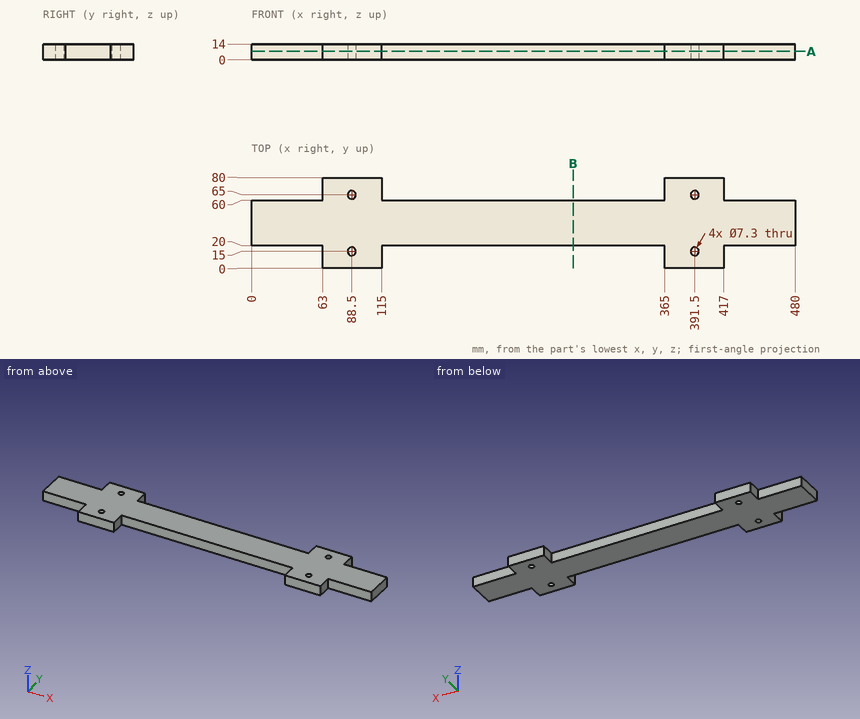
Geometry check sheet. Reference: drawing and pictorial views, mm from the part's lowest x, y, z. Round coordinates to 2 decimals unless told otherwise and drop trailing zeros. Order: outer loops, then holes, each group sorted by start corner. A loop starts at its lowest first (then second) coordinate and runs counter-clockwise, first axis right, second up. Notation, with made-up numbers: (21.25, -4) -> (31.25, -4) arc R29 ccw to (31.25, 25) -> close; hole circle Ø9 at (-0.75, -28). An arc over 180 degrees is marked (long way). One line per item, written item: value. Start each with the question number.
Q1. Gauge pin test, flat ends, axial feed: pin 1 Ø7 at (y, z) = (11.5, 4.5) entering from -X; pin 2 Ø11.5 at (x, y) = (391.5, 15) entering from +Z; pin 3 Ø2 at (x, z) = (215.5, 2) entering from -Y; pin 4 Ø7 at (y, z) = (14, 4) entering from +X. Record the tip position at first contact, or that the pin passes through.
Q2. Cross-section at A-A (z = 7.5). Record the boundary of the cut face in (x, y), and give its area (3 significant figures).
Q3. Thickness scan on line 1 (Y direction, x = 88.5, z = 11); line 2 (Y direction, x = 91, z = 8.75); line 3 (Y direction, x = 161, z = 4.25). Record the ranges inside material, lowest first.
Q4. Cross-section at B-B (x = 284). Record the boundary of the cut face in (y, z).
Completed:
1. pin 1: stops at x = 63
1. pin 2: stops at z = 14
1. pin 3: stops at y = 20
1. pin 4: stops at x = 417
2. outline: (0, 20) -> (63, 20) -> (63, 0) -> (115, 0) -> (115, 20) -> (365, 20) -> (365, 0) -> (417, 0) -> (417, 20) -> (480, 20) -> (480, 60) -> (417, 60) -> (417, 80) -> (365, 80) -> (365, 60) -> (115, 60) -> (115, 80) -> (63, 80) -> (63, 60) -> (0, 60) -> close; hole circle Ø7.3 at (88.5, 15); hole circle Ø7.3 at (88.5, 65); hole circle Ø7.3 at (391.5, 15); hole circle Ø7.3 at (391.5, 65)
2. area: 23,200 mm²
3. line 1: y = 0 to 11.35, 18.65 to 61.35, 68.65 to 80
3. line 2: y = 0 to 12.34, 17.66 to 62.34, 67.66 to 80
3. line 3: y = 20 to 60
4. outline: (20, 0) -> (60, 0) -> (60, 14) -> (20, 14) -> close
